For this review, use the dimensioned drawing (mm, ordinates from the lowest corner) and the shaded views. A direction names the side the tool comes from. Coordinates: 2 decimals unless noted, no trailing zeros. Loops run counter-clockwise (first coordinate to the right, second up) from the corner with the lowest first, then second, coordinate; pieces in that order, holes last. Notation, with made-up numbers: M -16.5,-18.5 L 39.5,-18.5 A37 ccw 39.5,18.5 Z; hole C 36,74.25 d5. An arc over 180 degrees is marked long. One line per item, written item: value.
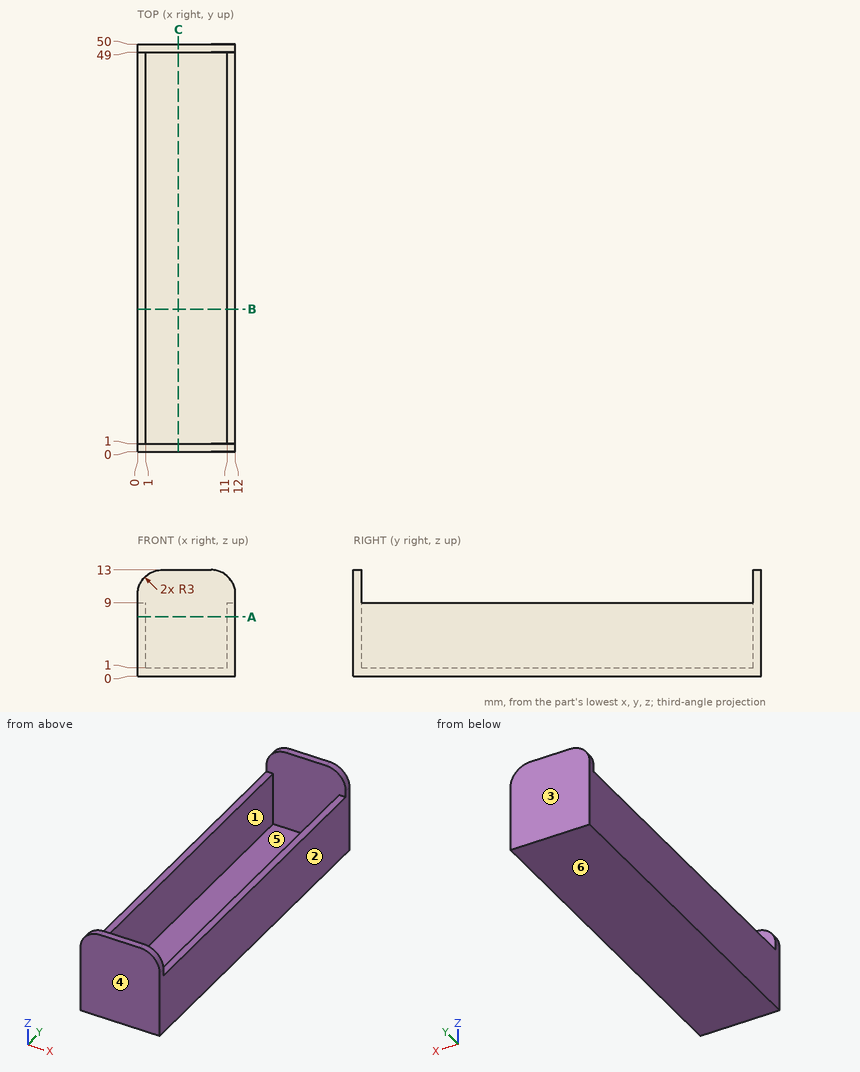
(1) Mouldability with a two-part tool opening along Y and no side actions: class the marked faces 1, 2, 3 and 4 as released by +Y, released by -Y, zero draft, split by the parting line, or undercut.
Reply:
face 1: undercut
face 2: zero draft
face 3: released by +Y
face 4: released by -Y
(2) We need section A-A on z = 7.25. State the section outline as (x, y) points.
Reply:
outline: M 0,0 L 12,0 L 12,50 L 0,50 Z; hole M 1,1 L 11,1 L 11,49 L 1,49 Z
(3) We need section B-B on y = 17.5. State the section outline as (x, z) points.
Reply:
outline: M 0,0 L 12,0 L 12,9 L 11,9 L 11,1 L 1,1 L 1,9 L 0,9 Z
(4) To check wall thickness, follow line 1 along X through (y, z) = (7, 3); line 2 along Y through (x, z) = (11.25, 9.25); line 3 along Z through (x, y) = (7, 19). State the ranges of each line that lie inside material, in increasing order. Write a range as [from, to].
Reply:
line 1: x = [0, 1], [11, 12]
line 2: y = [0, 1], [49, 50]
line 3: z = [0, 1]
(5) Insertion check: pin 1 (1 mm diameter, centred on x = 9, y = 18.5, fed in from +Z); pin 2 (0.8 mm diameter, centred on x = 11.5, y = 23, fed in from +Z). Each pin has a flat end and moves straight along its axis. Give the tip position at first contact, or say it passes through.
Reply:
pin 1: stops at z = 1
pin 2: stops at z = 9
(6) We need section C-C on x = 5. State the section outline as (y, z) points.
Reply:
outline: M 0,0 L 50,0 L 50,13 L 49,13 L 49,1 L 1,1 L 1,13 L 0,13 Z
(7) Tool access review of the marked faces 5 and 6: name each direction out of +Z, -Z, +X, -X, +Y, -Y from which nothing blocks a thin tool from reaching the whole face with its end or side.
Reply:
face 5: +Z
face 6: -Z, +X, -X, +Y, -Y
